from build123d import *

# Parameters (mm, degrees)
ESQUISSE2_R             = 35
BOSS_EXTRU_1_DEPTH      = 40
CONG_1_R                = 10
ESQUISSE3_R             = 25
ENL_V_MAT_EXTRU_1_DEPTH = 30
ENL_V_START             = -3
ESQUISSE7_R             = 25
ENL_V_MAT_EXTRU_3_DEPTH = 3
ESQUISSE8_R             = 10
ENL_V_MAT_EXTRU_4_DEPTH = 45
ESQUISSE4_R             = 2.5
ENL_V_MAT_EXTRU_5_DEPTH = 30


with BuildPart() as part:
    # Esquisse2 → Boss.-Extru.1 (new body)
    with BuildSketch(Plane(origin=(0, 0, 0), x_dir=(1, 0, 0), z_dir=(0, 1, 0))):
        with Locations(Location((0, 0, 0), (0, 0, 270))):
            Circle(ESQUISSE2_R)
    extrude(amount=BOSS_EXTRU_1_DEPTH)

    # Congé1
    cong_1_edges = [part.edges().sort_by_distance(p)[0] for p in [
        (0, 40, -35),
    ]]
    fillet(cong_1_edges, radius=CONG_1_R)

    # Esquisse3 → Enlèv. mat.-Extru.1 (cut)
    with BuildSketch(Plane.XZ):
        with Locations(Location((0, 0, 0), (0, 0, 270))):
            Circle(ESQUISSE3_R)
    extrude(amount=-ENL_V_MAT_EXTRU_1_DEPTH, mode=Mode.SUBTRACT)

    # Esquisse7 → Enlèv. mat.-Extru.3 (cut)
    with BuildSketch(Plane(origin=(0, 40, 0), x_dir=(1, 0, 0), z_dir=(0, 1, 0)).offset(ENL_V_START)):
        with Locations(Location((0, 0, 0), (0, 0, 90))):
            Circle(ESQUISSE7_R)
    extrude(amount=ENL_V_MAT_EXTRU_3_DEPTH, mode=Mode.SUBTRACT)

    # Esquisse8 → Enlèv. mat.-Extru.4 (cut)
    with BuildSketch(Plane.XY):
        with Locations(Location((0, 15, 0), (0, 0, 180))):
            Circle(ESQUISSE8_R)
    extrude(amount=ENL_V_MAT_EXTRU_4_DEPTH, mode=Mode.SUBTRACT)

    # Esquisse4 → Enlèv. mat.-Extru.5 (cut)
    with BuildSketch(Plane.XZ):
        with Locations((0, 25)):
            Circle(ESQUISSE4_R)
    extrude(amount=-ENL_V_MAT_EXTRU_5_DEPTH, mode=Mode.SUBTRACT)


solid = part.part
The listing builds one solid part. Answer for the finished solid, in the listing's coordinates (mm). A direction names the side the tool comes from. Round coordinates to 2 decimals unless told otherwise and drop trailing zeros. Order: outer loops, then holes, each group sorted by start corner. A loop starts at its lowest first (then second) coordinate and runs counter-clockwise, first axis right, second up. Notation, with made-up numbers: (9.25, 34.5) -> (45.25, 34.5) arc R38 ccw to (45.25, 73.5) -> close; hole circle Ø4 at (40, -7.75). An arc over 180 degrees is marked (long way). Put each result on its own line as item: value.
Q1. Section C-C, the plane y = 22.5 is taken. Write down the section's boundary in (x, z), and give its area (3 significant figures).
Results list:
outline: (-6.61, 24.11) -> (-6.61, 34.37) arc R35 ccw (long way) to (6.61, 34.37) -> (6.61, 24.11) arc R25 cw (long way) to start
area: 1,750 mm^2
Q2. Section A-A, the plane z = 0 is taken. Write down the section's boundary in (x, y), and give its area (3 significant figures).
Results list:
outline: (-35, 0) -> (-25, 0) -> (-25, 30) -> (25, 30) -> (25, 0) -> (35, 0) -> (35, 30) arc R10 ccw to (25, 40) -> (25, 37) -> (-25, 37) -> (-25, 40) arc R10 ccw to (-35, 30) -> close
area: 1,110 mm^2
Q3. Consider line 1 along X through (y, z) = (38, 0); line 2 along Z through (x, y) = (18.5, 29); line 3 along X through (y, z) = (26.5, -5). Determine where each line is inside the solid, lowest interval first.
Results list:
line 1: -31 to -25, 25 to 31
line 2: -29.71 to -16.82, 16.82 to 29.71
line 3: -34.64 to -24.49, 24.49 to 34.64
Q4. Section B-B, the plane y = 12.5 is taken. Write down the section's boundary in (x, z), and give its area (3 significant figures).
Results list:
outline: (-9.68, 23.05) -> (-9.68, 33.63) arc R35 ccw (long way) to (9.68, 33.63) -> (9.68, 23.05) arc R25 cw (long way) to start
area: 1,690 mm^2
Q5. Each of these flat-tipped pins is pushed along its axis until it touches: P1, Ø6, axis at y = 14.5, z = -10.5, coming from the -X side; P2, Ø8, axis at x = 9, z = 11.5, coming from the -Y side; P3, Ø4, axis at x = 25.5, z = 20, coming from the +Y side; P4, Ø1, axis at x = -22, z = -13.5, coming from the -Y side. Where does it stop, or does it pass through?
Results list:
P1: x = -34.19
P2: y = 30
P3: y = 38.41
P4: y = 0
Q6. Determine the mould class of faces 4 (the cylindrical face through (0.1, 2.6, 27.5)), 5 (the cylindrical face through (-21, 15, -28)), 6 (the flat face through (8, 0, -24)) for opening direction X: pulls with the +X half, pulls with the -X half, needs draft (parallel to the pull), parting line crosses it, or undercut.
Results list:
face 4: undercut
face 5: parting line crosses it
face 6: needs draft
Q7. Which of the six approach directions +Z, -Z, +X, -X, +Y, -Y give full straight-line access (tool end or side, diameter ignored) to faces 1 (the flat face through (0, 30, 2)), 2 (the cylindrical face through (-9.237, 18.83, 28.872)), 3 (the flat face through (0, 37, 0))?
Results list:
face 1: -Y
face 2: +Z
face 3: +Y
